Can you work these out from the drawing? Everything is in mm from the part's minimum corner. A direction names the side the tool comes from. Give positions to 0.01 mm unless a question says otherwise; leave off trailing zeros. Write each loop counter-clockwise with the first axis right and the second up, starting at its lowest first coordinate (ties: lowest second). Pieces come first, ordered by that corner, then holes. Notation, with made-up numbers: (86.5, -12) - (134.5, -12) arc R24 ccw to (134.5, 7) - close; hole circle Ø2 at (49, 21). An arc over 180 degrees is marked (long way). Use a Markdown table: item, result.
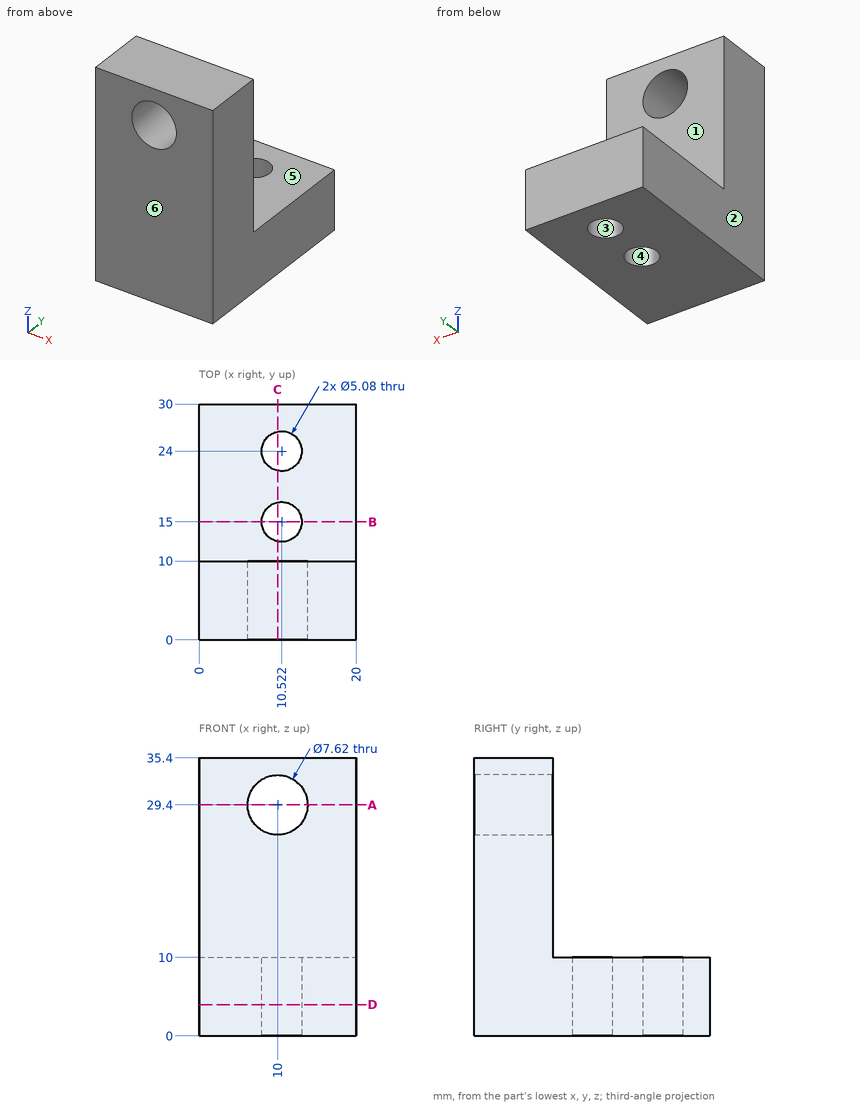
Item 1: If we section it at C-C, the plane x = 10: Write out the boundary of the cut face in (y, z).
Values:
| item | result |
|---|---|
| outline | (0, 0) - (12.51, 0) - (12.51, 10) - (10, 10) - (10, 25.59) - (0, 25.59) - close; (0, 33.21) - (10, 33.21) - (10, 35.4) - (0, 35.4) - close; (17.49, 0) - (21.51, 0) - (21.51, 10) - (17.49, 10) - close; (26.49, 0) - (30, 0) - (30, 10) - (26.49, 10) - close |
Item 2: If we section it at D-D, the plane z = 4: Write out the boundary of the cut face in (x, y).
Values:
| item | result |
|---|---|
| outline | (0, 0) - (20, 0) - (20, 30) - (0, 30) - close; hole circle Ø5.08 at (10.52, 15); hole circle Ø5.08 at (10.52, 24) |
Item 3: If we section it at A-A, the plane z = 29.4: Write out the boundary of the cut face in (x, y), plus the area to 3 significant figures.
Values:
| item | result |
|---|---|
| outline | (0, 0) - (6.19, 0) - (6.19, 10) - (0, 10) - close; (13.81, 0) - (20, 0) - (20, 10) - (13.81, 10) - close |
| area | 124 mm2 |
Item 4: Thinking about a two-plate mould opening in Y: for the marked faces 1, 2, 3 and 4, which applies, +Y half, -Y half, draft (parallel to the pull), parting line (faces both ways), or undercut?
Values:
| item | result |
|---|---|
| face 1 | +Y half |
| face 2 | draft |
| face 3 | undercut |
| face 4 | undercut |
Item 5: I need wall thicknesses on line 1 along Y through (x, z) = (10.75, 5); line 2 along X through (y, z) = (4.75, 29.4); line 3 along Y through (x, z) = (2, 21.5). Which ranges of each line are inside material? Lowest first, please. Write a range as [from, to].
Values:
| item | result |
|---|---|
| line 1 | y = [0, 12.47], [17.53, 21.47], [26.53, 30] |
| line 2 | x = [0, 6.19], [13.81, 20] |
| line 3 | y = [0, 10] |
Item 6: For the marked faces 5 and 6, which set-ups out of +Z, -Z, +X, -X, +Y, -Y let a thin tool reach every point of the face, with its end or its side?
Values:
| item | result |
|---|---|
| face 5 | +Z, +X, -X, +Y |
| face 6 | +Z, -Z, +X, -X, -Y |
Item 7: Will these pins go through, and if not, where does the flat tip stop? pin 1 Ø4.5 at (x, y) = (10.52, 24) entering from -Z (3 decimals); pin 2 Ø5 at (x, z) = (13.5, 20.5) entering from +Y; pin 3 Ø6 at (x, y) = (5, 19.5) entering from +Z; pin 4 Ø9 at (x, z) = (10, 29.4) entering from -Y.
Values:
| item | result |
|---|---|
| pin 1 | passes through |
| pin 2 | stops at y = 10 |
| pin 3 | stops at z = 10 |
| pin 4 | stops at y = 0 |
Item 8: If we section it at B-B, the plane y = 15: Write out the boundary of the cut face in (x, z).
Values:
| item | result |
|---|---|
| outline | (0, 0) - (7.98, 0) - (7.98, 10) - (0, 10) - close; (13.06, 0) - (20, 0) - (20, 10) - (13.06, 10) - close |
